```python
from build123d import *

# Parameters (mm, degrees)
EXTRUDE_1_DEPTH     = 15
SKETCH_2_R          = 1.5
CUT_EXTRUDE_1_DEPTH = 32.400636936
FILLET_1_R          = 1


with BuildPart() as part:
    # 草图1 → 凸台-拉伸1 (new body)
    with BuildSketch(Plane.XY):
        Polygon((20, 0), (-20, 0), (-20, 6), (-10, 6), (-10, 25), (10, 25), (10, 6), (20, 6), align=None)
    extrude(amount=EXTRUDE_1_DEPTH)

    # 草图2 → 切除-拉伸1 (cut, through all)
    with BuildSketch(Plane(origin=(0, 6, 0), x_dir=(1, 0, 0), z_dir=(0, 1, 0))):
        with Locations(Location((-15, -7.5, 0), (0, 0, 180))):
            Circle(SKETCH_2_R)
        with Locations((15, -7.5)):
            Circle(SKETCH_2_R)
    extrude(amount=-CUT_EXTRUDE_1_DEPTH, mode=Mode.SUBTRACT)

    # 圆角1
    fillet_1_edges = [part.edges().sort_by_distance(p)[0] for p in [
        (-10, 6, 7.5),
        (10, 6, 7.5),
    ]]
    fillet(fillet_1_edges, radius=FILLET_1_R)


solid = part.part
```
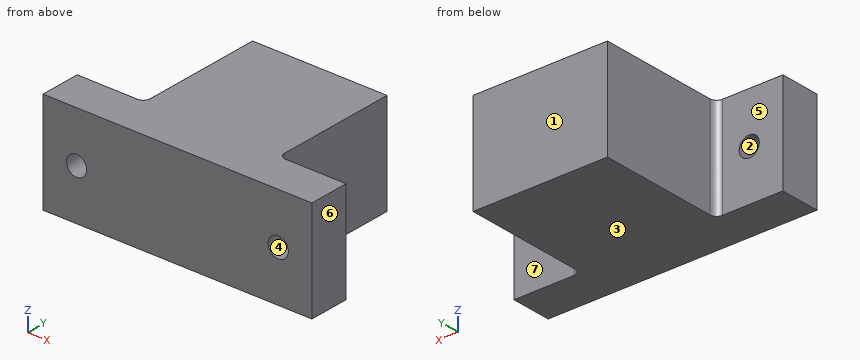
Geometry check sheet. Reference: the model listing, model coordinates, mm. Face numbers are marked on the shaded views. A direction names the side the tool comes from. Round coordinates to 2 decimals unless told otherwise and drop trailing zeros. Order: outer loops, then holes, each group sorted by start corner. A loop starts at its lowest first (then second) coordinate and runs counter-clockwise, first axis right, second up. Notation, with made-up numbers: (4.5, 53) - (10.5, 53) arc R18 cw to (10.5, 72) - close; hole circle Ø7 at (-9, 11.5). An arc over 180 degrees is marked (long way). Use a Markdown table: item, result. Add a question column.
(1) Depth check by flat-ended pin: pin 1 (4 mm diameter, centred on y = 13.5, z = 13, fed in from -X); pin 2 (1.5 mm diameter, centred on x = -11.5, z = 5, fed in from +Y); pin 3 (2.5 mm diameter, centred on x = 15, z = 7.5, fed in from +Y); pin 4 (4.5 mm diameter, centred on y = 15, z = 5, fed in from +X). Enter the tip coordinate at first touch or a pass-through.
(2) Sectioned sample at B-B, the plane z = 7.5. Enter the section's corners in (x, y), and give its area (3 significant figures).
(3) Sectioned sample at A-A, the plane x = -15. Enter the section's corners in (y, z), and give its area (3 significant figures).
(4) Material ranges on line 1 along Z through (x, y) = (15, 3.9); line 2 along Y through (x, z) = (18.5, 7); line 3 along X through (y, z) = (14.25, 8.5), recorded low to high. Write a range as [from, to].
(5) Sectioned sample at C-C, the plane y = 3. Enter the section's corners in (x, z), and give its area (3 significant figures).
(6) Release check for a two-part mould opening along Z. For the marked faces 1, 2, 3 and 4 record: pulls with the +Z half, pulls with the -Z half, needs draft (parallel to the pull), parting line crosses it, or undercut.
(7) Tool access check on the marked faces 5, 6 and 7. Record the directions out of +Z, -Z, +X, -X, +Y, -Y that give a thin tool (end or side, any length) a straight path to the whole face; none if there is none.
(8) Sectioned sample at D-D, the plane z = 3.5. Enter the section's corners in (x, y).
Answers below:
| question | item | result |
|---|---|---|
| 1 | pin 1 | x = -10 |
| 1 | pin 2 | y = 6.03 |
| 1 | pin 3 | through |
| 1 | pin 4 | x = 10 |
| 2 | outline | (-20, 0) - (-16.5, 0) - (-16.5, 6) - (-20, 6) - close; (-13.5, 0) - (13.5, 0) - (13.5, 6) - (11, 6) arc R1 cw to (10, 7) - (10, 25) - (-10, 25) - (-10, 7) arc R1 cw to (-11, 6) - (-13.5, 6) - close; (16.5, 0) - (20, 0) - (20, 6) - (16.5, 6) - close |
| 2 | area | 584 mm² |
| 3 | outline | (0, 0) - (6, 0) - (6, 6) - (0, 6) - close; (0, 9) - (6, 9) - (6, 15) - (0, 15) - close |
| 3 | area | 72.0 mm² |
| 4 | line 1 | [0, 6], [9, 15] |
| 4 | line 2 | [0, 6] |
| 4 | line 3 | [-10, 10] |
| 5 | outline | (-20, 0) - (20, 0) - (20, 15) - (-20, 15) - close; hole circle Ø3 at (-15, 7.5); hole circle Ø3 at (15, 7.5) |
| 5 | area | 586 mm² |
| 6 | face 1 | needs draft |
| 6 | face 2 | undercut |
| 6 | face 3 | pulls with the -Z half |
| 6 | face 4 | undercut |
| 7 | face 5 | +Z, -Z, -X, +Y |
| 7 | face 6 | +Z, -Z, +X, +Y, -Y |
| 7 | face 7 | +Z, -Z, +X, +Y |
| 8 | outline | (-20, 0) - (20, 0) - (20, 6) - (11, 6) arc R1 cw to (10, 7) - (10, 25) - (-10, 25) - (-10, 7) arc R1 cw to (-11, 6) - (-20, 6) - close |
